Check sheet for the modelled part. Datum: model origin and axes. Units: mm. Coordinates: 2 decimals unless noted, no trailing zeros. Loops run counter-clockwise (first coordinate to the right, second up) from the corner with the lowest first, then second, coordinate; pieces in that order, holes last. Notation, with made-up numbers: M -21,52 L 21,52 A35 cw 21,88 Z; hole C 57.25,-38.5 d4. An arc over 180 degrees is marked long. Return JSON: item names as keys, results as strings.
from build123d import *

# Parameters (mm, degrees)
SKETCH1_W           = 40
SKETCH1_H           = 160
BOSS_EXTRUDE1_DEPTH = 3.175
SKETCH2_W           = 3.175
SKETCH2_H           = 10
SKETCH2_H_2         = 20
CUT_EXTRUDE1_DEPTH  = 3.175
SKETCH3_R           = 1
CUT_EXTRUDE2_DEPTH  = 3.175
SKETCH4_W           = 20
SKETCH4_H           = 3.175
CUT_EXTRUDE3_DEPTH  = 3.175
SKETCH5_R           = 3.5
CUT_EXTRUDE4_DEPTH  = 3.175


with BuildPart() as part:
    # Sketch1 → Boss-Extrude1 (new body)
    with BuildSketch(Plane(origin=(0, 0, -55.956765442), x_dir=(-1, 0, 0), z_dir=(0, 0, -1))):
        with Locations((-25.376465458, 105.316281379)):
            Rectangle(SKETCH1_W, SKETCH1_H)
    extrude(amount=-BOSS_EXTRUDE1_DEPTH)

    # Sketch2 → Cut-Extrude1 (cut)
    with BuildSketch(Plane(origin=(0, 0, -55.956765442), x_dir=(-1, 0, 0), z_dir=(0, 0, -1))):
        with Locations((-6.963965458, 180.316281379)):
            Rectangle(SKETCH2_W, SKETCH2_H)
        with Locations((-6.963965458, 145.316281379)):
            Rectangle(SKETCH2_W, SKETCH2_H_2)
        with Locations((-6.963965458, 105.316281379)):
            Rectangle(SKETCH2_W, SKETCH2_H_2)
        with Locations((-6.963965458, 65.316281379)):
            Rectangle(SKETCH2_W, SKETCH2_H_2)
        with Locations((-6.963965458, 30.316281379)):
            Rectangle(SKETCH2_W, SKETCH2_H)
    cut_extrude1 = extrude(amount=-CUT_EXTRUDE1_DEPTH, mode=Mode.SUBTRACT)

    # Sketch3 → Cut-Extrude2 (cut)
    with BuildSketch(Plane(origin=(0, 0, -55.956765442), x_dir=(-1, 0, 0), z_dir=(0, 0, -1))):
        with Locations((-23.551465458, 32.666436233)):
            Circle(SKETCH3_R)
        with Locations((-23.551465458, 49.666436233)):
            Circle(SKETCH3_R)
    cut_extrude2 = extrude(amount=-CUT_EXTRUDE2_DEPTH, mode=Mode.SUBTRACT)

    # Mirror1: Cut-Extrude1 across plane
    add(cut_extrude1.mirror(Plane.ZY.offset(-25.376465458)), mode=Mode.SUBTRACT)

    # Sketch4 → Cut-Extrude3 (cut)
    with BuildSketch(Plane(origin=(0, 0, -55.956765442), x_dir=(-1, 0, 0), z_dir=(0, 0, -1))):
        with Locations((-25.376465458, 26.903781379)):
            Rectangle(SKETCH4_W, SKETCH4_H)
        with Locations((-25.376465458, 183.728781379)):
            Rectangle(SKETCH4_W, SKETCH4_H)
    extrude(amount=-CUT_EXTRUDE3_DEPTH, mode=Mode.SUBTRACT)

    # Sketch5 → Cut-Extrude4 (cut)
    with BuildSketch(Plane(origin=(0, 0, -55.956765442), x_dir=(-1, 0, 0), z_dir=(0, 0, -1))):
        with Locations((-23.551465458, 41.425244037)):
            Circle(SKETCH5_R)
    cut_extrude4 = extrude(amount=-CUT_EXTRUDE4_DEPTH, mode=Mode.SUBTRACT)

    # Mirror2: Cut-Extrude2, Cut-Extrude4 across plane
    add(cut_extrude2.mirror(Plane(origin=(0, 105.316281379, 0), x_dir=(0, 0, 1), z_dir=(0, -1, 0))), mode=Mode.SUBTRACT)
    add(cut_extrude4.mirror(Plane(origin=(0, 105.316281379, 0), x_dir=(0, 0, 1), z_dir=(0, -1, 0))), mode=Mode.SUBTRACT)


solid = part.part
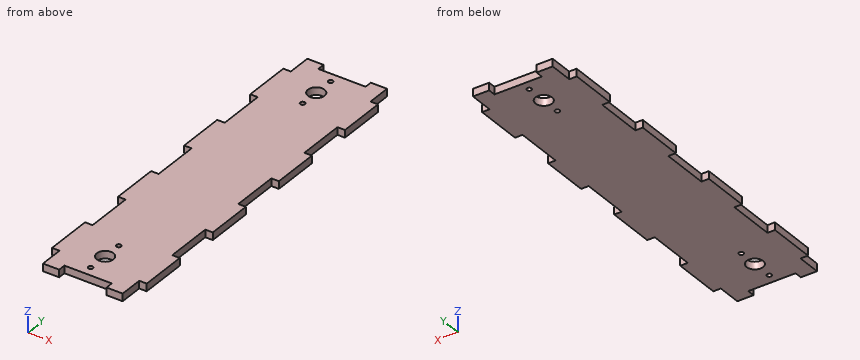
1) Section check B-B on y = 99.5. Record the cut outline in (x, z), then the cut area to 3 significant figures.
Answers:
{"outline": "M 8.55,-55.96 L 42.2,-55.96 L 42.2,-52.78 L 8.55,-52.78 Z", "area": "107 mm²"}
2) Scan lines: line 1 along Y through (x, z) = (8, -55.65); line 2 along X through (y, z) = (41, -55.2); line 3 along X through (y, z) = (74.5, -53.45). Record each from-to range of solid material in increasing order. Write a range as [from, to].
Answers:
{"line 1": "[35.32, 55.32], [75.32, 95.32], [115.32, 135.32], [155.32, 175.32]", "line 2": "[5.38, 20.08], [27.03, 45.38]", "line 3": "[8.55, 42.2]"}
3) Go/stop test with flat-tipped pins: pin 1 Ø2.5 at (x, y) = (23.55, 49.67) entering from -Z; pin 2 Ø1 at (y, z) = (63, -54) entering from -X; pin 3 Ø1.6 at (y, z) = (184.5, -53.5) entering from +X; pin 4 Ø1.6 at (x, z) = (43.5, -54) entering from +Y. Record where each tip stops, or that it passes through.
Answers:
{"pin 1": "z = -55.96", "pin 2": "x = 8.55", "pin 3": "x = 42.2", "pin 4": "y = 175.32"}
4) Section check A-A on x = 33.5. Record the cut outline in (y, z).
Answers:
{"outline": "M 28.49,-55.96 L 182.14,-55.96 L 182.14,-52.78 L 28.49,-52.78 Z"}
5) Section check C-C on z = -54.8. Count the separate pieces of the cut face and the enclosed holes in it, then the cut area to 3 significant figures.
Answers:
{"separate pieces": "1", "enclosed holes": "6", "area": "5,680 mm²"}
